```python
from build123d import *

# Parameters (mm, degrees)
SKETCH_1_W      = 47
SKETCH_1_H      = 79.13
SKETCH_1_W_2    = 37
SKETCH_1_H_2    = 70.13
EXTRUDE_2_DEPTH = 10
SKETCH_2_W      = 15.5
SKETCH_2_H      = 6
SKETCH_2_R      = 1
EXTRUDE_3_DEPTH = 5
EXTRUDE_START   = -42
SKETCH_2_2_W    = 15.5
SKETCH_2_2_H    = 6
SKETCH_2_2_R    = 1
EXTRUDE_4_DEPTH = 5


with BuildPart() as part:
    # 스케치1 → 보스-돌출2 (new body)
    # profile 1 of 8: a face of its own
    with BuildSketch(Plane.XY):
        with Locations((3.5, -0.384376544)):
            Rectangle(SKETCH_1_W, SKETCH_1_H)
        with Locations((3.5, 0.115623456)):
            Rectangle(SKETCH_1_W_2, SKETCH_1_H_2, mode=Mode.SUBTRACT)
    # profile 2 of 8: a face of its own
    with BuildSketch(Plane.XY):
        Polygon((-10.329391215, 35.180623456), (-15, 35.180623456), (-15, 32.967449172), (17.329391215, 17.648123456), (22, 19.861297741), align=None)
    # profile 3 of 8: a face of its own
    with BuildSketch(Plane.XY):
        Polygon((22, 15.434949172), (22, 19.861297741), (17.329391215, 17.648123456), align=None)
    # profile 4 of 8: a face of its own
    with BuildSketch(Plane.XY):
        Polygon((17.329391215, 17.648123456), (-15, 2.328797741), (-10.329391215, 0.115623456), (22, 15.434949172), align=None)
    # profile 5 of 8: a face of its own
    with BuildSketch(Plane.XY):
        Polygon((-10.329391215, 0.115623456), (-15, 2.328797741), (-15, -2.097550828), align=None)
    # profile 6 of 8: a face of its own
    with BuildSketch(Plane.XY):
        Polygon((-10.329391215, 0.115623456), (-15, -2.097550828), (17.329391215, -17.416876544), (22, -15.203702259), align=None)
    # profile 7 of 8: a face of its own
    with BuildSketch(Plane.XY):
        Polygon((22, -19.630050828), (22, -15.203702259), (17.329391215, -17.416876544), align=None)
    # profile 8 of 8: a face of its own
    with BuildSketch(Plane.XY):
        Polygon((17.329391215, -17.416876544), (-15, -32.736202259), (-15, -34.949376544), (-10.329391215, -34.949376544), (22, -19.630050828), align=None)
    extrude(amount=EXTRUDE_2_DEPTH)

    # 스케치2 → 보스-돌출3 (add)
    # profile 1 of 4: a face of its own
    with BuildSketch(Plane(origin=(27, 0, 0), x_dir=(0, 0, -1), z_dir=(1, 0, 0))):
        with Locations((-17.75, -36.949376544)):
            Rectangle(SKETCH_2_W, SKETCH_2_H)
        with Locations(Location((-20.333333333, -37.449376544, 0), (0, 0, 90))):
            Circle(SKETCH_2_R, mode=Mode.SUBTRACT)
        with Locations(Location((-15.166666667, -37.449376544, 0), (0, 0, 90))):
            Circle(SKETCH_2_R, mode=Mode.SUBTRACT)
    # profile 2 of 4: a face of its own
    with BuildSketch(Plane(origin=(27, 0, 0), x_dir=(0, 0, -1), z_dir=(1, 0, 0))):
        with Locations((7.75, -36.949376544)):
            Rectangle(SKETCH_2_W, SKETCH_2_H)
        with Locations(Location((5.166666667, -37.449376544, 0), (0, 0, 90))):
            Circle(SKETCH_2_R, mode=Mode.SUBTRACT)
        with Locations(Location((10.333333333, -37.449376544, 0), (0, 0, 90))):
            Circle(SKETCH_2_R, mode=Mode.SUBTRACT)
    # profile 3 of 4: a face of its own
    with BuildSketch(Plane(origin=(27, 0, 0), x_dir=(0, 0, -1), z_dir=(1, 0, 0))):
        with Locations((-17.75, 2.110623456)):
            Rectangle(SKETCH_2_W, SKETCH_2_H)
        with Locations(Location((-20.333333333, 2.110623456, 0), (0, 0, 90))):
            Circle(SKETCH_2_R, mode=Mode.SUBTRACT)
        with Locations(Location((-15.166666667, 2.110623456, 0), (0, 0, 90))):
            Circle(SKETCH_2_R, mode=Mode.SUBTRACT)
    # profile 4 of 4: a face of its own
    with BuildSketch(Plane(origin=(27, 0, 0), x_dir=(0, 0, -1), z_dir=(1, 0, 0))):
        with Locations((7.75, 2.110623456)):
            Rectangle(SKETCH_2_W, SKETCH_2_H)
        with Locations(Location((5.166666667, 2.110623456, 0), (0, 0, 90))):
            Circle(SKETCH_2_R, mode=Mode.SUBTRACT)
        with Locations(Location((10.333333333, 2.110623456, 0), (0, 0, 90))):
            Circle(SKETCH_2_R, mode=Mode.SUBTRACT)
    extrude(amount=-EXTRUDE_3_DEPTH)

    # 스케치2<2> → 보스-돌출4 (add)
    # profile 1 of 4: a face of its own
    with BuildSketch(Plane(origin=(27, 0, 0), x_dir=(0, 0, -1), z_dir=(1, 0, 0)).offset(EXTRUDE_START)):
        with Locations((-17.75, -36.949376544)):
            Rectangle(SKETCH_2_2_W, SKETCH_2_2_H)
        with Locations(Location((-20.333333333, -37.449376544, 0), (0, 0, 90))):
            Circle(SKETCH_2_2_R, mode=Mode.SUBTRACT)
        with Locations(Location((-15.166666667, -37.449376544, 0), (0, 0, 90))):
            Circle(SKETCH_2_2_R, mode=Mode.SUBTRACT)
    # profile 2 of 4: a face of its own
    with BuildSketch(Plane(origin=(27, 0, 0), x_dir=(0, 0, -1), z_dir=(1, 0, 0)).offset(EXTRUDE_START)):
        with Locations((7.75, -36.949376544)):
            Rectangle(SKETCH_2_2_W, SKETCH_2_2_H)
        with Locations(Location((5.166666667, -37.449376544, 0), (0, 0, 90))):
            Circle(SKETCH_2_2_R, mode=Mode.SUBTRACT)
        with Locations(Location((10.333333333, -37.449376544, 0), (0, 0, 90))):
            Circle(SKETCH_2_2_R, mode=Mode.SUBTRACT)
    # profile 3 of 4: a face of its own
    with BuildSketch(Plane(origin=(27, 0, 0), x_dir=(0, 0, -1), z_dir=(1, 0, 0)).offset(EXTRUDE_START)):
        with Locations((-17.75, 2.110623456)):
            Rectangle(SKETCH_2_2_W, SKETCH_2_2_H)
        with Locations(Location((-20.333333333, 2.110623456, 0), (0, 0, 90))):
            Circle(SKETCH_2_2_R, mode=Mode.SUBTRACT)
        with Locations(Location((-15.166666667, 2.110623456, 0), (0, 0, 90))):
            Circle(SKETCH_2_2_R, mode=Mode.SUBTRACT)
    # profile 4 of 4: a face of its own
    with BuildSketch(Plane(origin=(27, 0, 0), x_dir=(0, 0, -1), z_dir=(1, 0, 0)).offset(EXTRUDE_START)):
        with Locations((7.75, 2.110623456)):
            Rectangle(SKETCH_2_2_W, SKETCH_2_2_H)
        with Locations(Location((5.166666667, 2.110623456, 0), (0, 0, 90))):
            Circle(SKETCH_2_2_R, mode=Mode.SUBTRACT)
        with Locations(Location((10.333333333, 2.110623456, 0), (0, 0, 90))):
            Circle(SKETCH_2_2_R, mode=Mode.SUBTRACT)
    extrude(amount=-EXTRUDE_4_DEPTH)


solid = part.part
```
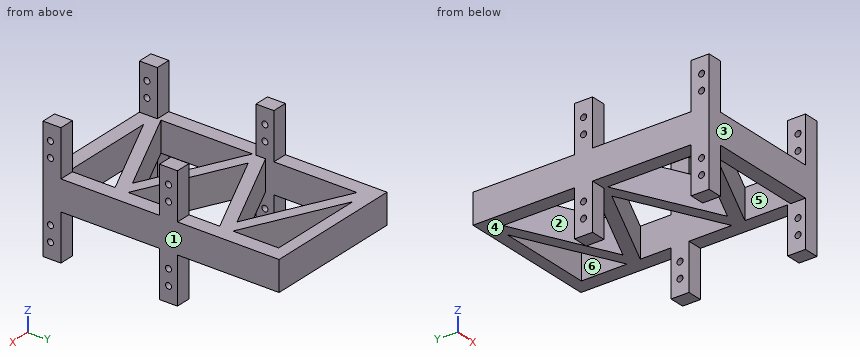
Here's how the part is built. I have some questions about the finished solid (model axes, mm). Face numbers are marked on the shaded views. A direction names the side the tool comes from. Give positions to 0.01 mm unless a question says otherwise; leave off trailing zeros. Order: outer loops, then holes, each group sorted by start corner. A loop starts at its lowest first (then second) coordinate and runs counter-clockwise, first axis right, second up. Notation, with made-up numbers: M 67.25,34 L 77.25,34 A14 ccw 77.25,44 Z; hole C 83,18 d7. An arc over 180 degrees is marked long. Use a Markdown table: item, result. Add a question column.
1. Suppose I cut it at B-B (x = -7.5). List the corners of the cut face in (y, z) for me.
2. Suppose I cut it at A-A (z = 7). List the corners of the cut face in (x, y) for me.
3. Suppose I cut it at C-C (y = -8). List the corners of the cut face in (x, z) for me.
4. On a 3-axis mill with a long thin cutter (end or side, diameter ignored), from which of +Z, -Z, +X, -X, +Y, -Y can I reach the whole of each face in a straight line? I mean the marked faces 4, 5 and 6. Say none if no direction works.
5. I need wall thicknesses on probe 1 along Y at (x, z) = (-17.5, 13.5); probe 2 along Y at (x, z) = (4.5, 6.5); probe 3 along X at (y, z) = (-12, 4.5). Which ranges of each line are inside material? Lowest first, please. Write a range as from..to.
6. For pin 1 Ø12 at (x, y) = (-8, 23.5) entering from +Z; pin 2 Ø1.5 at (x, z) = (-16.5, -8.5) entering from +Y; pin 3 Ø14 at (x, y) = (-2, -5) entering from -Z, each with a flat end and sliding along its axis, tell me the tip position at first contact or that it passes through.
7. Suppose I cut it at D-D (x = 19). List the corners of the cut face in (y, z) for me.
8. If we mould it in two halves opening along Y, with no side actions, what happens to the marked faces 1, 2 and 3? For each: +Y half, -Y half, draft (parallel to the pull), parting line (faces both ways), or undercut.
Results list:
| question | item | result |
|---|---|---|
| 1 | outline | M -39.95,0 L -34.95,0 L -34.95,10 L -39.95,10 Z; M -33.61,0 L -29.18,0 L -29.18,10 L -33.61,10 Z; M -5.65,0 L -1.23,0 L -1.23,10 L -5.65,10 Z; M 1.46,0 L 5.88,0 L 5.88,10 L 1.46,10 Z; M 29.41,0 L 33.84,0 L 33.84,10 L 29.41,10 Z; M 35.18,0 L 39.18,0 L 39.18,10 L 35.18,10 Z |
| 2 | outline | M -20,-39.95 L 27,-39.95 L 27,39.18 L -20,39.18 Z; hole M -15,-32.74 L 17.33,-17.42 L -15,-2.1 Z; hole M -15,2.33 L 17.33,17.65 L -15,32.97 Z; hole M -10.33,-34.95 L 22,-34.95 L 22,-19.63 Z; hole M -10.33,0.12 L 22,-15.2 L 22,15.43 Z; hole M -10.33,35.18 L 22,19.86 L 22,35.18 Z |
| 3 | outline | M -20,0 L -15,0 L -15,10 L -20,10 Z; M -2.54,0 L 6.8,0 L 6.8,10 L -2.54,10 Z; M 22,0 L 27,0 L 27,10 L 22,10 Z |
| 4 | face 4 | -Z |
| 4 | face 5 | none |
| 4 | face 6 | +Z, -Z |
| 5 | probe 1 | y = -39.95..-33.95, -0.89..5.11 |
| 5 | probe 2 | y = -39.95..-34.95, -27.92..-23.5, -11.34..-6.91, 7.14..11.57, 23.73..28.15, 35.18..39.18 |
| 5 | probe 3 | x = -20..-15, 5.9..15.24, 22..27 |
| 6 | pin 1 | stops at z = 10 |
| 6 | pin 2 | stops at y = 5.11 |
| 6 | pin 3 | stops at z = 0 |
| 7 | outline | M -39.95,0 L -34.95,0 L -34.95,10 L -39.95,10 Z; M -21.05,0 L -13.78,0 L -13.78,10 L -21.05,10 Z; M 14.01,0 L 21.28,0 L 21.28,10 L 14.01,10 Z; M 35.18,0 L 39.18,0 L 39.18,10 L 35.18,10 Z |
| 8 | face 1 | draft |
| 8 | face 2 | undercut |
| 8 | face 3 | -Y half |
